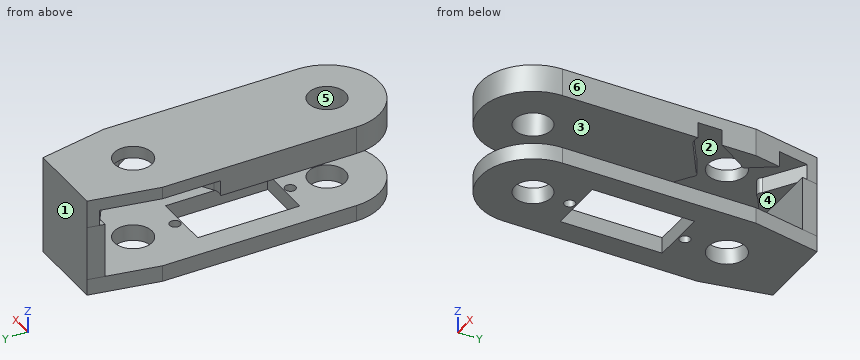
```python
from build123d import *

# Parameters (mm, degrees)
SKETCH1_R              = 4.572
SKETCH1_R_2            = 4.445
BOSS_EXTRUDE1_DEPTH    = 6.731
BOSS_EXTRUDE3_START    = -13.208
SKETCH1_5_R            = 4.572
SKETCH1_5_R_2          = 1.2954
SKETCH1_5_R_3          = 4.445
SKETCH1_5_W            = 13.97
SKETCH1_5_H            = 24.765
BOSS_EXTRUDE3_DEPTH    = 3.937
CUT_EXTRUDE4_START     = -3.81
CUT_EXTRUDE4_OUTLINE_R = 4.572
CUT_EXTRUDE4_DEPTH     = 3.81
BOSS_EXTRUDE5_DEPTH    = 16.4211


# Read off the part's stored shape, not the designer's step: Cut-Extrude4
with BuildPart() as part:
    # Sketch1 (on Front Plane) → Boss-Extrude1 (new body)
    with BuildSketch(Plane.XY):
        with BuildLine():
            Line((-12.7, 0), (-9.525, 16.51))
            Line((-9.525, 16.51), (9.525, 16.51))
            Line((9.525, 16.51), (12.7, 0))
            Line((12.7, 0), (12.7, -46.99))
            ThreePointArc((12.7, -46.99), (0, -59.69), (-12.7, -46.99))
            Line((-12.7, -46.99), (-12.7, 0))
        make_face()
        Circle(SKETCH1_R, mode=Mode.SUBTRACT)
        with Locations((0, -46.99)):
            Circle(SKETCH1_R_2, mode=Mode.SUBTRACT)
    extrude(amount=BOSS_EXTRUDE1_DEPTH)

    # Cut-Extrude4 outline → Cut-Extrude4 (cut)
    with BuildSketch(Plane(origin=(0, 0, 0), x_dir=(-1, 0, 0), z_dir=(0, 0, -1)).offset(CUT_EXTRUDE4_START)):
        with BuildLine():
            Line((1.021082558, -8.023816422), (10.113003756, -13.894226547))
            ThreePointArc((10.113003756, -13.894226547), (11.380658922, -14.323016968), (12.7, -14.099075092))
            Line((12.7, -14.099075092), (12.7, 0))
            Line((12.7, 0), (10.037418608, 13.84542324))
            Line((10.037418608, 13.84542324), (1.021082558, 8.023816422))
            ThreePointArc((1.021082558, 8.023816422), (0, 7.408645479), (-1.021082558, 8.023816422))
            Line((-1.021082558, 8.023816422), (-10.037418608, 13.84542324))
            Line((-10.037418608, 13.84542324), (-11.47556666, 6.367053366))
            Line((-11.47556666, 6.367053366), (-8.023816422, 1.021082558))
            ThreePointArc((-8.023816422, 1.021082558), (-7.408645479, 0), (-8.023816422, -1.021082558))
            Line((-8.023816422, -1.021082558), (-12.7, -8.263420264))
            Line((-12.7, -8.263420264), (-12.7, -14.099075092))
            ThreePointArc((-12.7, -14.099075092), (-11.380658922, -14.323016968), (-10.113003756, -13.894226547))
            Line((-10.113003756, -13.894226547), (-1.021082558, -8.023816422))
            ThreePointArc((-1.021082558, -8.023816422), (0, -7.408645479), (1.021082558, -8.023816422))
        make_face()
        Circle(CUT_EXTRUDE4_OUTLINE_R, mode=Mode.SUBTRACT)
    extrude(amount=CUT_EXTRUDE4_DEPTH, mode=Mode.SUBTRACT)



with BuildPart() as body_2:
    # Sketch1<5> → Boss-Extrude3 (new body)
    with BuildSketch(Plane.XY.offset(BOSS_EXTRUDE3_START)):
        with BuildLine():
            Line((-12.7, 0), (-9.525, 16.51))
            Line((-9.525, 16.51), (9.525, 16.51))
            Line((9.525, 16.51), (12.7, 0))
            Line((12.7, 0), (12.7, -46.99))
            ThreePointArc((12.7, -46.99), (0, -59.69), (-12.7, -46.99))
            Line((-12.7, -46.99), (-12.7, 0))
        make_face()
        Circle(SKETCH1_5_R, mode=Mode.SUBTRACT)
        with Locations((0, -10.16)):
            Circle(SKETCH1_5_R_2, mode=Mode.SUBTRACT)
        with Locations((0, -38.1)):
            Circle(SKETCH1_5_R_2, mode=Mode.SUBTRACT)
        with Locations((0, -46.99)):
            Circle(SKETCH1_5_R_3, mode=Mode.SUBTRACT)
        with Locations((0, -24.13)):
            Rectangle(SKETCH1_5_W, SKETCH1_5_H, mode=Mode.SUBTRACT)
    extrude(amount=-BOSS_EXTRUDE3_DEPTH)


with BuildPart() as part_1:
    add(part.part)

    add(body_2.part)  # Boss-Extrude5 merges body 2
    # Sketch5 → Boss-Extrude5 (add)
    with BuildSketch(Plane(origin=(0, 0, 0), x_dir=(-1, 0, 0), z_dir=(0, 0, -1))):
        Polygon((-9.525, 16.51), (9.525, 16.51), (10.282115385, 12.573), (-10.282115385, 12.573), align=None)
    extrude(amount=BOSS_EXTRUDE5_DEPTH)


solid = part_1.part
```
The model under review builds one solid part; all positions refer to its coordinate system, in mm. Face numbers are marked on the shaded views. A direction names the side the tool comes from. Round coordinates to 2 decimals unless told otherwise and drop trailing zeros. Order: outer loops, then holes, each group sorted by start corner. A loop starts at its lowest first (then second) coordinate and runs counter-clockwise, first axis right, second up. Notation, with made-up numbers: (14, -10.75) -> (61, -10.75) arc R19 ccw to (61, 24.25) -> close; hole circle Ø5 at (80, 84.5). An arc over 180 degrees is marked (long way). Use a Markdown table: item, result.
Q1. We need section B-B on z = 2.5. Write out the cut boundary in (x, y) (3 decimals).
Values:
| item | result |
|---|---|
| outline | (-12.7, -46.99) arc R12.7 ccw to (12.7, -46.99) -> (12.7, -14.099) arc R2.735 cw to (10.113, -13.894) -> (1.021, -8.024) arc R1.155 ccw to (-1.021, -8.024) -> (-10.113, -13.894) arc R2.735 cw to (-12.7, -14.099) -> close; (-10.037, 13.845) -> (-1.021, 8.024) arc R1.155 ccw to (1.021, 8.024) -> (10.037, 13.845) -> (9.525, 16.51) -> (-9.525, 16.51) -> close; (8.024, -1.021) -> (12.7, -8.263) -> (12.7, 0) -> (11.476, 6.367) -> (8.024, 1.021) arc R1.155 ccw to start; hole circle Ø8.89 at (0, -46.99) |
Q2. Mouldability with a two-part tool opening along X and no side actions: class the marked faces 4, 5 and 6 as +X half, -X half, draft (parallel to the pull), parting line (faces both ways), or undercut.
Values:
| item | result |
|---|---|
| face 4 | draft |
| face 5 | undercut |
| face 6 | +X half |
Q3. Tool access review of the marked faces 1, 2 and 3: name each direction out of +Z, -Z, +X, -X, +Y, -Y from which nothing blocks a thin tool from reaching the whole face with its end or side.
Values:
| item | result |
|---|---|
| face 1 | +Z, -Z, +X, -X, +Y |
| face 2 | none |
| face 3 | +X, -X, -Y |
Q4. We need section D-D on x = 0. State how many separate pieces and enclosed holes the cut face has, then the cut area to 3 significant figures.
Values:
| item | result |
|---|---|
| separate pieces | 8 |
| enclosed holes | 0 |
| area | 533 mm^2 |
Q5. We need section A-A on y = -16.5. Write out the cut boundary in (x, z) (3 decimals).
Values:
| item | result |
|---|---|
| outline | (-12.7, -17.145) -> (-6.985, -17.145) -> (-6.985, -13.208) -> (-12.7, -13.208) -> close; (-12.7, 0) -> (12.7, 0) -> (12.7, 6.731) -> (-12.7, 6.731) -> close; (6.985, -17.145) -> (12.7, -17.145) -> (12.7, -13.208) -> (6.985, -13.208) -> close |
Q6. We need section C-C on y = -45.5. Write out the cut boundary in (x, z) (3 decimals).
Values:
| item | result |
|---|---|
| outline | (-12.7, -17.145) -> (-4.188, -17.145) -> (-4.188, -13.208) -> (-12.7, -13.208) -> close; (-12.7, 0) -> (-4.188, 0) -> (-4.188, 6.731) -> (-12.7, 6.731) -> close; (4.188, -17.145) -> (12.7, -17.145) -> (12.7, -13.208) -> (4.188, -13.208) -> close; (4.188, 0) -> (12.7, 0) -> (12.7, 6.731) -> (4.188, 6.731) -> close |
Q7. Clearance check with flat-ended pins moving along their axes: P1, Ø5.5, axis at x = 0, y = -46.99, coming from the +Z side; P2, Ø3, axis at x = 3, z = -15.5, coming from the -Y side. State where each tip first meets the part, or that it passes through.
Values:
| item | result |
|---|---|
| P1 | passes through |
| P2 | stops at y = -59.6 |
Q8. For line 1 (Y direction, x = 0, z = -15.6) (1 decimal); line 2 (Z direction, x = 7.25, y = -33.5) (3 decimals); line 3 (Z direction, x = -11.25, y = 2) (3 decimals), list the stretches that pass through material, from the lowest coordinate up.
Values:
| item | result |
|---|---|
| line 1 | y = -59.7 to -51.4, -42.5 to -39.4, -36.8 to -36.5, -11.7 to -11.5, -8.9 to -4.6, 4.6 to 16.5 |
| line 2 | z = -17.145 to -13.208, 0 to 6.731 |
| line 3 | z = -17.145 to -13.208, 3.81 to 6.731 |
